from build123d import *

# Parameters (mm, degrees)
BOSS_EXTRUDE1_DEPTH      = 40
BOSS_EXTRUDE2_DEPTH      = 65
BOSS_EXTRUDE2_DEPTH_BACK = 105
SKETCH2_R                = 9
SKETCH3_W                = 15
SKETCH3_H                = 130
CUT_EXTRUDE1_DEPTH       = 31.813269935
SKETCH4_R                = 12
BOSS_EXTRUDE3_DEPTH      = 40
SKETCH5_R                = 26
BOSS_EXTRUDE4_DEPTH      = 15
SKETCH6_R                = 26
BOSS_EXTRUDE5_DEPTH      = 15


with BuildPart() as part:
    # Sketch1 → Boss-Extrude1 (new body)
    with BuildSketch(Plane(origin=(0, 0, 0), x_dir=(0, 0, -1), z_dir=(1, 0, 0))):
        with BuildLine():
            Line((-15.906634967, -42.094880497), (-15.906634967, 42.094880497))
            ThreePointArc((-15.906634967, 42.094880497), (0, 45), (15.906634967, 42.094880497))
            Line((15.906634967, 42.094880497), (15.906634967, -42.094880497))
            ThreePointArc((15.906634967, -42.094880497), (0, -45), (-15.906634967, -42.094880497))
        make_face()
    extrude(amount=BOSS_EXTRUDE1_DEPTH)

    # Sketch2 → Boss-Extrude2 (add, two sides: drawn at the far end of the back side and taken through both)
    with BuildSketch(Plane.ZY.offset(-BOSS_EXTRUDE2_DEPTH_BACK)):
        Circle(SKETCH2_R)
    extrude(amount=BOSS_EXTRUDE2_DEPTH + BOSS_EXTRUDE2_DEPTH_BACK)

    # Sketch3 → Cut-Extrude1 (cut)
    with BuildSketch(Plane.XY.offset(15.906634967)):
        with Locations((20, 0.729141458)):
            Rectangle(SKETCH3_W, SKETCH3_H)
    extrude(amount=-CUT_EXTRUDE1_DEPTH, mode=Mode.SUBTRACT)


with BuildPart() as cut_extrude1_piece_1:
    # of the separate pieces the step leaves, piece 1, a body of its own (cut_extrude1_pieces)
    add(part.part.solids().sort_by_distance((0, -42.094880497, -15.906634967))[0])



with BuildPart() as cut_extrude1_piece_2:
    # of the separate pieces the step leaves, piece 2, a body of its own (cut_extrude1_pieces)
    add(part.part.solids().sort_by_distance((27.5, -42.094880497, -15.906634968))[0])


with BuildPart() as cut_extrude1_piece_1_1:
    add(cut_extrude1_piece_1.part)

    add(cut_extrude1_piece_2.part)  # Boss-Extrude3 merges Cut-Extrude1 piece 2
    # Sketch4 → Boss-Extrude3 (add)
    with BuildSketch(Plane(origin=(40, 0, 0), x_dir=(0, 0, -1), z_dir=(1, 0, 0))):
        with Locations(Location((0, 25, 0), (0, 0, 90))):
            Circle(SKETCH4_R)
    extrude(amount=-BOSS_EXTRUDE3_DEPTH)

    # Sketch5 → Boss-Extrude4 (add)
    with BuildSketch(Plane.ZY):
        with Locations(Location((0, 0, 0), (0, 0, 127.719309026))):
            Circle(SKETCH5_R)
    extrude(amount=BOSS_EXTRUDE4_DEPTH)

    # Sketch6 → Boss-Extrude5 (add)
    with BuildSketch(Plane(origin=(40, 0, 0), x_dir=(0, 0, -1), z_dir=(1, 0, 0))):
        with Locations(Location((0, 0, 0), (0, 0, 52.280690974))):
            Circle(SKETCH6_R)
    extrude(amount=BOSS_EXTRUDE5_DEPTH)


solid = cut_extrude1_piece_1_1.part
Verification items for the finished model (mm, model axes). A direction names the side the tool comes from. Round coordinates to 2 decimals unless told otherwise and drop trailing zeros. Loops run counter-clockwise (first coordinate to the right, second up) from the corner with the lowest first, then second, coordinate; pieces in that order, holes last. Notation, with made-up numbers: (-2.5, 15) - (40.5, 15) arc R18 ccw to (40.5, 19) - close; hole circle Ø1 at (-23.75, 79.5). An arc over 180 degrees is marked (long way). Use a Markdown table: item, result. Add a question column.
1. Gauge pin test, flat ends, axial feed: pin 1 (6 mm diameter, centred on x = 3.5, y = 11, fed in from -Z); pin 2 (7.5 mm diameter, centred on y = 38.5, z = 0.5, fed in from +X); pin 3 (1.5 mm diameter, centred on x = -28.5, z = -7, fed in from +Y). Record the tip position at first contact, or that the pin passes through.
2. Section check B-B, the plane z = 0. Record the boundary of the cut face in (x, y), plus the area to 3 significant figures.
3. Section check A-A, the plane y = 0. Record the boundary of the cut face in (x, z), plus the area to 3 significant figures.
4. Section check C-C, the plane y = 15. Record the boundary of the cut face in (x, z).
5. Thickness scan on probe 1 along X at (y, z) = (-19, -15); probe 2 along X at (y, z) = (15.5, -16); probe 3 along Z at (x, y) = (36.5, 9). Record the ranges inside material, lowest first. Write a range as [from, to].
6. Access from +Z, -Z, +X, -X, +Y, -Y to the whole of each face (thin tool, end or side, straight path). Record for faces 1 (the face through (55, 9, -7)), 2 (the face through (20.105, 36.085, -4.596)), 3 (the face through (0, 1, -21)).
Checks:
| question | item | result |
|---|---|---|
| 1 | pin 1 | stops at z = -15.91 |
| 1 | pin 2 | stops at x = 40 |
| 1 | pin 3 | stops at y = 6.48 |
| 2 | outline | (-65, -9) - (-15, -9) - (-15, -26) - (0, -26) - (0, -45) - (12.5, -45) - (12.5, 13) - (27.5, 13) - (27.5, -45) - (40, -45) - (40, -26) - (55, -26) - (55, -9) - (105, -9) - (105, 9) - (55, 9) - (55, 26) - (40, 26) - (40, 45) - (27.5, 45) - (27.5, 37) - (12.5, 37) - (12.5, 45) - (0, 45) - (0, 26) - (-15, 26) - (-15, 9) - (-65, 9) - close |
| 2 | area | 5,970 mm^2 |
| 3 | outline | (-65, -9) - (-15, -9) - (-15, -26) - (0, -26) - (0, -15.91) - (12.5, -15.91) - (12.5, 15.91) - (0, 15.91) - (0, 26) - (-15, 26) - (-15, 9) - (-65, 9) - close; (27.5, -15.91) - (40, -15.91) - (40, -26) - (55, -26) - (55, -9) - (105, -9) - (105, 9) - (55, 9) - (55, 26) - (40, 26) - (40, 15.91) - (27.5, 15.91) - close |
| 3 | area | 4,160 mm^2 |
| 4 | outline | (-15, -21.24) - (0, -21.24) - (0, -15.91) - (12.5, -15.91) - (12.5, -6.63) - (27.5, -6.63) - (27.5, -15.91) - (40, -15.91) - (40, -21.24) - (55, -21.24) - (55, 21.24) - (40, 21.24) - (40, 15.91) - (27.5, 15.91) - (27.5, 6.63) - (12.5, 6.63) - (12.5, 15.91) - (0, 15.91) - (0, 21.24) - (-15, 21.24) - close |
| 5 | probe 1 | x = [-15, 12.5], [27.5, 55] |
| 5 | probe 2 | x = [-15, 0], [40, 55] |
| 5 | probe 3 | z = [-15.91, 15.91] |
| 6 | face 1 | +X |
| 6 | face 2 | none |
| 6 | face 3 | -Z, +Y, -Y |
